Design review of the part shown in the three views and the two pictorial views. Dimensions are in mm from the part's minimum x, y and z. Coordinates: 2 decimals unless noted, no trailing zeros. Loops run counter-clockwise (first coordinate to the right, second up) from the corner with the lowest first, then second, coordinate; pieces in that order, holes last. Notation, with made-up numbers: (40, -29.75) - (79, -29.75) arc R12 ccw to (79, -11.75) - close; hole circle Ø7 at (-30, 79.5). An arc over 180 degrees is marked (long way). One line per question, with ' | ' between items.
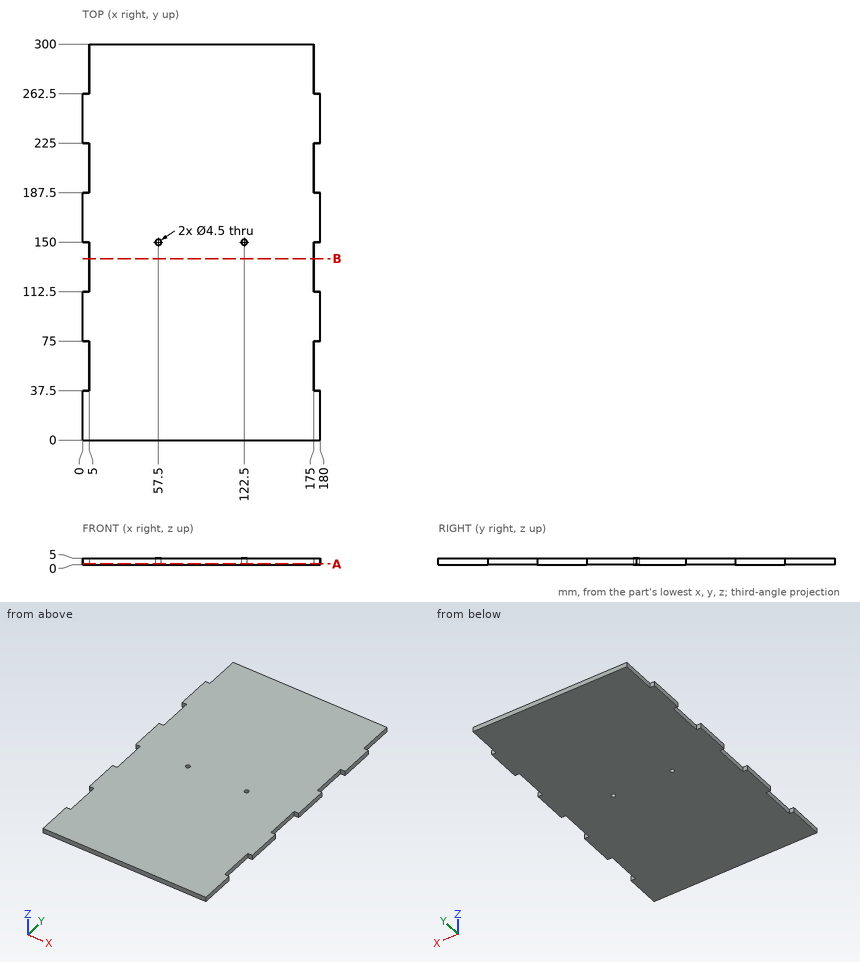
Q1. Take a section at A-A (z = 0.75). State how many separate pieces and enclosed holes the cut face has, plus the area to 3 significant figures.
Returned:
separate pieces: 1 | enclosed holes: 2 | area: 52,500 mm²
Q2. Take a section at B-B (y = 137.5). Give the boundary of the cut face in (x, z).
Returned:
outline: (5, 0) - (175, 0) - (175, 5) - (5, 5) - close
Q3. For pin 1 (2.5 mm diameter, centred on y = 54, z = 1.5, fed in from +X); pin 2 (2.5 mm diameter, centred on y = 138, z = 1.5, fed in from -X); pin 3 (2.5 mm diameter, centred on x = 178.5, z = 1.5, fed in from +Y); pin 4 (1.5 mm diameter, centred on x = 130, z = 4, fed in from -Y), all flat-tipped, find the tip position at first contact; note any pin that passes through.
Returned:
pin 1: stops at x = 175 | pin 2: stops at x = 5 | pin 3: stops at y = 262.5 | pin 4: stops at y = 0
Q4. To check wall thickness, follow line 1 along Y through (x, z) = (122.5, 1.7); line 2 along X through (y, z) = (206.5, 3.75). State the ranges of each line that lie inside material, in increasing order.
Returned:
line 1: y = 0 to 147.75, 152.25 to 300 | line 2: x = 5 to 175
